Read the model definition and answer for the solid it produces. Units are mm, in the model's axes. A direction names the side the tool comes from. Coordinates: 2 decimals unless noted, no trailing zeros. Loops run counter-clockwise (first coordinate to the right, second up) from the corner with the lowest first, then second, coordinate; pieces in that order, holes last. Notation, with made-up numbers: (-39.75, 64) -> (-8.75, 64) arc R19 ccw to (-8.75, 88) -> close; hole circle Ø8 at (-29, 69). An arc over 180 degrees is marked (long way). Answer as CSV lines item,"result".
```python
from build123d import *

# Parameters (mm, degrees)
SKETCH1_W           = 10.455425194
SKETCH1_H           = 3
SKETCH1_W_2         = 10
BOSS_EXTRUDE1_DEPTH = 2
SKETCH2_R           = 1
CUT_EXTRUDE2_DEPTH  = 47.542938032
BOSS_EXTRUDE3_DEPTH = 29
SKETCH3_W           = 33
SKETCH3_H           = 33
BOSS_EXTRUDE4_DEPTH = 2
SKETCH4_R           = 1.5
CUT_EXTRUDE4_DEPTH  = 58.019690289


with BuildPart() as part:
    # Sketch1 → Boss-Extrude1 (new body)
    with BuildSketch(Plane(origin=(0, 0, 0), x_dir=(1, 0, 0), z_dir=(0, 1, 0))):
        Polygon((-37.532221957, -24.451364186), (-14.987647151, -24.451364186), (-4.532221957, -24.451364186), (-4.532221957, 8.548635814), (-14.532221957, 8.548635814), (-37.532221957, 8.548635814), align=None)
        with Locations((-9.759934554, -25.951364186)):
            Rectangle(SKETCH1_W, SKETCH1_H)
        with Locations((-9.532221957, 10.048635814)):
            Rectangle(SKETCH1_W_2, SKETCH1_H)
    extrude(amount=BOSS_EXTRUDE1_DEPTH)

    # Sketch2 → Cut-Extrude2 (cut, through all)
    with BuildSketch(Plane(origin=(0, 2, 0), x_dir=(1, 0, 0), z_dir=(0, 1, 0))):
        with Locations(Location((-9.532221957, 7.548635814, 0), (0, 0, 270))):
            Circle(SKETCH2_R)
        with Locations(Location((-9.532221957, -23.451364186, 0), (0, 0, 270))):
            Circle(SKETCH2_R)
    extrude(amount=-CUT_EXTRUDE2_DEPTH, mode=Mode.SUBTRACT)

    # 3DSketch1 → Boss-Extrude3 (add)
    with BuildSketch(Plane(origin=(-37.532221957, 2, 22.951364186), x_dir=(0.589695128953028, 0, -0.8076259374791475), z_dir=(0, -1, 0))):
        Polygon((0, 0), (-1.211438906, 0.884542693), (12.35154906, 19.459939255), (13.562987966, 18.575396562), align=None)
        Polygon((39.003204997, 0), (37.79176609, 0.884542693), (24.228778124, -17.690853869), (25.440217031, -18.575396562), align=None)
    extrude(amount=-BOSS_EXTRUDE3_DEPTH)

    # Sketch3 → Boss-Extrude4 (add)
    with BuildSketch(Plane(origin=(0, 31, 0), x_dir=(1, 0, 0), z_dir=(0, 1, 0))):
        with Locations((-21.032221957, -7.951364186)):
            Rectangle(SKETCH3_W, SKETCH3_H)
    extrude(amount=BOSS_EXTRUDE4_DEPTH)

    # Sketch4 → Cut-Extrude4 (cut, through all)
    with BuildSketch(Plane(origin=(0, 33, 0), x_dir=(1, 0, 0), z_dir=(0, 1, 0))):
        with Locations(Location((-8.532221957, -17.951364186, 0), (0, 0, 270))):
            Circle(SKETCH4_R)
        with Locations(Location((-8.532221957, 2.048635814, 0), (0, 0, 270))):
            Circle(SKETCH4_R)
        with Locations(Location((-33.532221957, -7.951364186, 0), (0, 0, 270))):
            Circle(SKETCH4_R)
    extrude(amount=-CUT_EXTRUDE4_DEPTH, mode=Mode.SUBTRACT)


solid = part.part
```
Q1. A cutting plane is placed at D-D, the plane z = 25.5. Write down the section's boundary in (x, y).
Results:
outline,"(-14.99, 0) -> (-4.53, 0) -> (-4.53, 2) -> (-14.99, 2) -> close"
Q2. For faces 4 (the face through (-10, 1, -11.549)), 5 (the face through (-14.532, 1, -10)), 6 (the face through (-26, 16, -7.049)), 7 (the face through (-14.988, 1, 26)), 8 (the face through (-4.532, 32, 8)), determine the directions among +Z, -Z, +X, -X, +Y, -Y from which every point of the face is accessible in a straight line to the end or side of a thin tool.
Results:
face 4,"-Z, +X, -X, +Y, -Y"
face 5,"-Z, -X, +Y, -Y"
face 6,"+X, -X"
face 7,"+Z, -X, +Y, -Y"
face 8,"+Z, -Z, +X, +Y, -Y"
Q3. Find the intervals of material crossed by probe 1 along Y at (x, z) = (-33, -2); probe 2 along Z at (x, y) = (-26.5, 28.5); probe 3 along X at (y, z) = (8, 24), in increasing order. Write a range as [from, to].
Results:
probe 1,"y = [0, 2], [31, 33]"
probe 2,"z = [-8.55, -7.05], [22.95, 24.45]"
probe 3,"x = [-37.53, -14.53]"
Q4. For a pull along X with two mould halves and no side action, classify faces 1 (the face through (-21, 31, 8)), 2 (the face through (-14.532, 16, 24)), 3 (the face through (-9.488, 1.014, -8.548)) as pulls with the +X half, pulls with the -X half, needs draft (parallel to the pull), parting line crosses it, or undercut.
Results:
face 1,"needs draft"
face 2,"pulls with the +X half"
face 3,"undercut"
Q5. A cutting plane is placed at B-B, the plane y = 18.5. Write down the section's boundary in (x, z), and give its area (3 significant figures).
Results:
outline,"(-37.53, -8.55) -> (-14.53, -8.55) -> (-14.53, -7.05) -> (-37.53, -7.05) -> close; (-37.53, 22.95) -> (-14.53, 22.95) -> (-14.53, 24.45) -> (-37.53, 24.45) -> close"
area,"69.0 mm²"
Q6. A cutting plane is placed at A-A, the plane x = -11.5. Write down the section's boundary in (y, z), and give its area (3 significant figures).
Results:
outline,"(0, -11.55) -> (2, -11.55) -> (2, 27.45) -> (0, 27.45) -> close; (31, -8.55) -> (33, -8.55) -> (33, 24.45) -> (31, 24.45) -> close"
area,"144 mm²"
Q7. A cutting plane is placed at C-C, the plane x = -24. Write down the section's boundary in (y, z).
Results:
outline,"(0, -8.55) -> (33, -8.55) -> (33, 24.45) -> (0, 24.45) -> close; hole (2, -7.05) -> (31, -7.05) -> (31, 22.95) -> (2, 22.95) -> close"
Q8. Given pin 1 Ø18.5 at (x, y) = (-31, 17.5) entering from -Z; pin 2 Ø1.6 at (x, y) = (-28, 1.5) entering from +Z; pin 3 Ø3.5 at (x, z) = (-8.53, 17.95) entering from +Y; pin 4 Ø0.6 at (y, z) = (1, 26.5) entering from -X, each flat-ended and moving along its own axis, determine where each tip first touches the part or whether it passes through.
Results:
pin 1,"stops at z = -8.55"
pin 2,"stops at z = 24.45"
pin 3,"stops at y = 33"
pin 4,"stops at x = -14.99"
